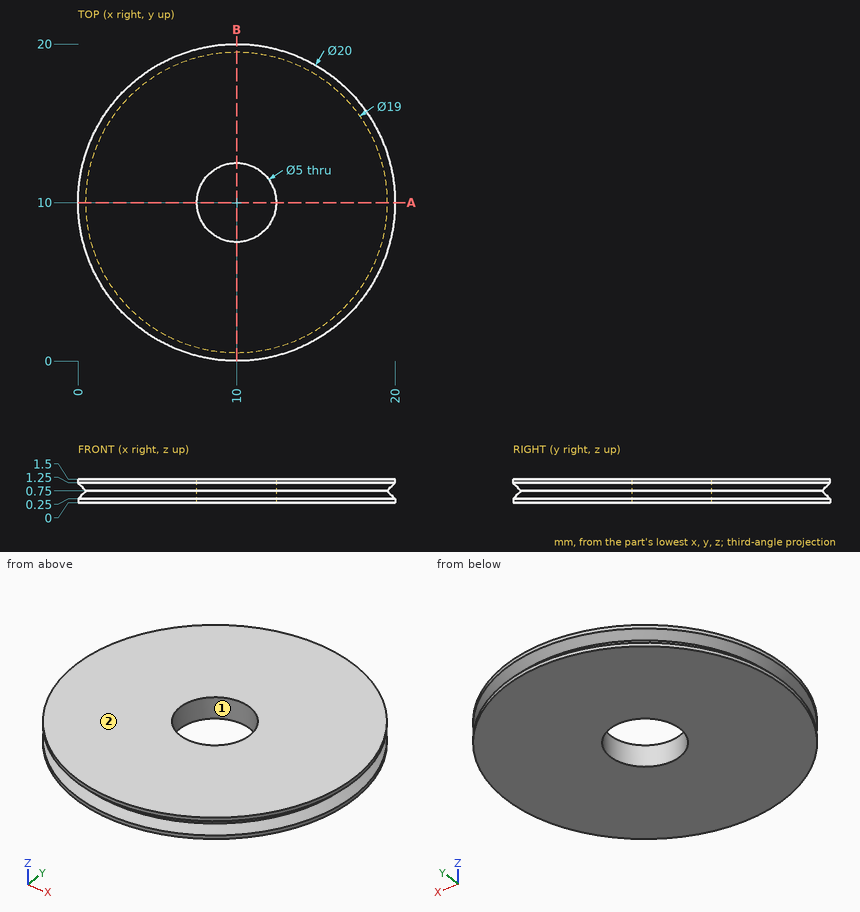
Geometry: see drawing. Coordinates: mm, zero at the bounding-box minimum. Give positions to 0.01 mm unless a question says otherwise; leave off trailing zeros. Loops run counter-clockwise (first coordinate to the right, second up) from the corner with the lowest first, then second, coordinate; pieces in that order, holes last. Notation, with made-up numbers: (-7.5, -20.75) - (35.5, -20.75) arc R21 cw to (35.5, -7.75) - close; hole circle Ø9 at (82, -24). An arc over 180 degrees is marked (long way). Use CSV: the item, a comma, the result in double quotes. Start each with the question number.
Item 1: Line query: line 1 (Z direction, x = 1, y = 6.5); line 2 (Y direction, x = 10, z = 0.9); line 3 (Y direction, x = 10, z = 0.55). Output: solid intervals per line, ascending.
Item 2: Mould query, pull axis X, two halves, no side actions, for the marked faces 1 and 2. Classes: pulls with the +X half, pulls with the -X half, needs draft (parallel to the pull), parting line crosses it, or undercut.
Item 3: Section A-A on y = 10. Return loops of the section in (x, z).
Ans:
1,line 1,"z = 0 to 0.59, 0.91 to 1.5"
1,line 2,"y = 0.35 to 7.5, 12.5 to 19.65"
1,line 3,"y = 0.3 to 7.5, 12.5 to 19.7"
2,face 1,"undercut"
2,face 2,"needs draft"
3,outline,"(0, 0) - (7.5, 0) - (7.5, 1.5) - (0, 1.5) - (0, 1.25) - (0.5, 0.75) - (0, 0.25) - close; (12.5, 0) - (20, 0) - (20, 0.25) - (19.5, 0.75) - (20, 1.25) - (20, 1.5) - (12.5, 1.5) - close"
